Check sheet for the modelled part. Datum: model origin and axes. Units: mm. Face numbers are marked on the shaded views. Give positions to 0.01 mm unless a question says otherwise; leave off trailing zeros. Loops run counter-clockwise (first coordinate to the right, second up) from the corner with the lowest first, then second, coordinate; pieces in that order, holes last. Notation, with made-up numbers: (37, 84) -> (91, 84) arc R15 ccw to (91, 106) -> close; hole circle Ø3 at (48, 46.5). An arc over 180 degrees is marked (long way). Answer as CSV lines item,"result". Start each with the question number.
(1) Material ranges on line 1 (Y direction, x = -6.45, z = 0.6); line 2 (Y direction, x = -6.45, z = 5.5); line 3 (X direction, y = 16.5, z = 3), recorded low to high. Write a range as from..to.
(2) Section check D-D on y = 5.25. Enter the section's corners in (x, z).
(3) Section check A-A on y = 57.75. Enter the section's corners in (x, z).
(4) Section check C-C on x = -10. Enter the section's corners in (y, z).
(5) Section check B-B on x = -6.45. Enter the section's corners in (y, z).
(6) Release check for a two-part mould opening along Y. For the marked faces 1, 2 and 3 record: pulls with the +Y half, pulls with the -Y half, needs draft (parallel to the pull), parting line crosses it, or undercut.
(7) Gauge pin test, flat ends, axial feed: pin 1 Ø0.5 at (y, z) = (10, 1) entering from -X; pin 2 Ø2 at (y, z) = (31, 5) entering from +X; pin 3 Ø4 at (x, z) = (-8.5, 5.5) entering from +Y. Record the tip position at first contact, or that the pin passes through.
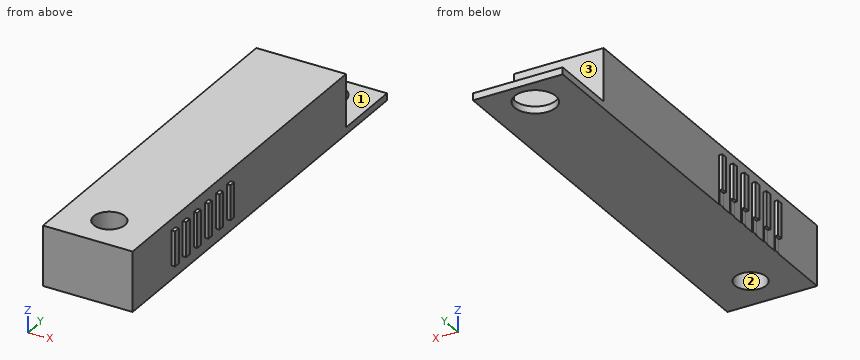
Autodesk Fusion 360 part; units mm, degrees
sketch "Sketch1" plane through (0, 0, 0) normal (0, 0, 1) x (1, 0, 0)
  line L0 (0, 0) -> (-12.9, 0)
  line L1 (-12.9, 0) -> (-12.9, 62)
  line L2 (-12.9, 62) -> (0, 62)
  line L3 (0, 62) -> (0, 0)
  circle A0 centre (-6.45, 57.75) radius 2.95
  line L4 (-12.9, 62) -> (0, 62)
  line L5 (0, 62) -> (0, 52)
  line L6 (0, 52) -> (-12.9, 52)
  line L7 (-12.9, 52) -> (-12.9, 62)
  line L8 (-12.9, 9.5) -> (-13.4, 9.5)
  line L9 (-13.4, 9.5) -> (-13.4, 10.4)
  line L10 (-13.4, 10.4) -> (-12.9, 10.4)
  line L11 (-12.9, 10.4) -> (-12.9, 9.5)
  line L12 (-12.9, 13.1) -> (-13.4, 13.1)
  line L13 (-13.4, 13.1) -> (-13.4, 12.2)
  line L14 (-13.4, 12.2) -> (-12.9, 12.2)
  line L15 (-12.9, 12.2) -> (-12.9, 13.1)
  line L16 (-12.9, 14.9) -> (-13.4, 14.9)
  line L17 (-13.4, 14.9) -> (-13.4, 15.8)
  line L18 (-13.4, 15.8) -> (-12.9, 15.8)
  line L19 (-12.9, 15.8) -> (-12.9, 14.9)
  line L20 (-12.9, 17.6) -> (-13.4, 17.6)
  line L21 (-13.4, 17.6) -> (-13.4, 18.5)
  line L22 (-13.4, 18.5) -> (-12.9, 18.5)
  line L23 (-12.9, 18.5) -> (-12.9, 17.6)
  line L24 (-12.9, 20.3) -> (-13.4, 20.3)
  line L25 (-13.4, 20.3) -> (-13.4, 21.2)
  line L26 (-13.4, 21.2) -> (-12.9, 21.2)
  line L27 (-12.9, 21.2) -> (-12.9, 20.3)
  line L28 (-12.9, 23) -> (-13.4, 23)
  line L29 (-13.4, 23) -> (-13.4, 23.9)
  line L30 (-13.4, 23.9) -> (-12.9, 23.9)
  line L31 (-12.9, 23.9) -> (-12.9, 23)
  line L32 (0.5, 23.9) -> (0, 23.9)
  line L33 (0.5, 23) -> (0.5, 23.9)
  line L34 (0, 23) -> (0.5, 23)
  line L35 (0.5, 21.2) -> (0, 21.2)
  line L36 (0.5, 20.3) -> (0.5, 21.2)
  line L37 (0, 20.3) -> (0.5, 20.3)
  line L38 (0.5, 18.5) -> (0, 18.5)
  line L39 (0.5, 17.6) -> (0.5, 18.5)
  line L40 (0, 17.6) -> (0.5, 17.6)
  line L41 (0.5, 15.8) -> (0, 15.8)
  line L42 (0.5, 14.9) -> (0.5, 15.8)
  line L43 (0, 14.9) -> (0.5, 14.9)
  line L44 (0, 13.1) -> (0.5, 13.1)
  line L45 (0.5, 13.1) -> (0.5, 12.2)
  line L46 (0.5, 12.2) -> (0, 12.2)
  line L47 (0.5, 10.4) -> (0, 10.4)
  line L48 (0.5, 9.5) -> (0.5, 10.4)
  line L49 (0, 9.5) -> (0.5, 9.5)
  circle A1 centre (-6.45, 5.25) radius 2.25
  dimension "d1" = 12.9
  dimension "d2" = 62
  dimension "d3" = 5.9
  dimension "d4" = 4.25
  dimension "d5" = 6.45
  dimension "d6" = 10
  dimension "d7" = 0.5
  dimension "d8" = 0.9
  dimension "d9" = 9.5
  dimension "d10" = 0.5
  dimension "d11" = 0.9
  dimension "d12" = 0.5
  dimension "d13" = 0.9
  dimension "d14" = 0.5
  dimension "d15" = 0.9
  dimension "d16" = 0.9
  dimension "d17" = 0.5
  dimension "d18" = 0.9
  dimension "d19" = 1.8
  dimension "d20" = 2.7
  dimension "d21" = 1.8
  dimension "d22" = 1.8
  dimension "d23" = 1.8
  dimension "d24" = 4.5
  dimension "d25" = 5.25
  dimension "d26" = 6.45
extrude "Extrude1" add sketch "Sketch1" along normal blind 1 contours L1 L2 L3 L4 L5 L6 L7
extrude "Extrude2" add sketch "Sketch1" along normal blind 8.6 contours L0 L1 L3 L6 L11 L15 L19 L23 L27 L31
extrude "Extrude3" add sketch "Sketch1" along normal blind 7 contours L3 L47 L48 L49 | L1 L8 L9 L10 L11 | L3 L44 L45 L46 | L1 L12 L13 L14 L15 | L3 L41 L42 L43 | L1 L16 L17 L18 L19 | L3 L38 L39 L40 | L1 L20 L21 L22 L23 | L3 L35 L36 L37 | L1 L24 L25 L26 L27 | L3 L32 L33 L34 | L1 L28 L29 L30 L31
sketch "Sketch2" plane through (0, 0, 0) normal (0, 0, 1) x (1, 0, 0)
  line L0 (0, 0) -> (22, 0)
  line L1 (22, 0) -> (22, 28)
  line L2 (22, 28) -> (0, 28)
  line L3 (0, 28) -> (0, 0)
  line L4 (-13, 0) -> (-34, 0)
  line L5 (-34, 0) -> (-34, 25)
  line L6 (-34, 25) -> (-13, 25)
  line L7 (-13, 25) -> (-13, 0)
extrude "Extrude4" cut sketch "Sketch2" along normal blind 2
equation "d4 = d3 / 2 + 1.3 mm"
equation "d5 = d3 / 2 + ( d1 - d3 ) / 2"
equation "d20 = 1.8 mm + d13"
equation "d25 = d24 / 2 + 3 mm"
equation "d26 = d24 / 2 + ( d1 - d24 ) / 2"
Working result:
1,line 1,"y = 0..3, 7.5..54.8, 60.7..62"
1,line 2,"y = 0..3, 7.5..52"
1,line 3,"x = -12.9..0"
2,outline,"(-12.9, 0) -> (-8.7, 0) -> (-8.7, 8.6) -> (-12.9, 8.6) -> close; (-4.2, 0) -> (0, 0) -> (0, 8.6) -> (-4.2, 8.6) -> close"
3,outline,"(-12.9, 0) -> (-9.4, 0) -> (-9.4, 1) -> (-12.9, 1) -> close; (-3.5, 0) -> (0, 0) -> (0, 1) -> (-3.5, 1) -> close"
4,outline,"(0, 0) -> (62, 0) -> (62, 1) -> (52, 1) -> (52, 8.6) -> (0, 8.6) -> close"
5,outline,"(0, 0) -> (3, 0) -> (3, 8.6) -> (0, 8.6) -> close; (7.5, 0) -> (54.8, 0) -> (54.8, 1) -> (52, 1) -> (52, 8.6) -> (7.5, 8.6) -> close; (60.7, 0) -> (62, 0) -> (62, 1) -> (60.7, 1) -> close"
6,face 1,"needs draft"
6,face 2,"undercut"
6,face 3,"pulls with the +Y half"
7,pin 1,"stops at x = -13"
7,pin 2,"stops at x = 0"
7,pin 3,"stops at y = 52"
